from build123d import *

# Parameters (mm, degrees)
SKETCH1_W           = 105
SKETCH1_H           = 60
BOSS_EXTRUDE1_DEPTH = 15
SHELL1_T            = 2.5
FILLET1_R           = 2.5
SKETCH3_R           = 1.5
BOSS_EXTRUDE2_DEPTH = 3
SKETCH4_W           = 2
SKETCH4_H           = 60
BOSS_EXTRUDE3_DEPTH = 10
BOSS_EXTRUDE4_DEPTH = 6
SKETCH7_W           = 9
SKETCH7_H           = 10
CUT_EXTRUDE1_DEPTH  = 2.5


with BuildPart() as part:
    # Sketch1 → Boss-Extrude1 (new body)
    with BuildSketch(Plane(origin=(0, 0, 0), x_dir=(1, 0, 0), z_dir=(0, 1, 0))):
        Rectangle(SKETCH1_W, SKETCH1_H)
    extrude(amount=BOSS_EXTRUDE1_DEPTH)

    # Shell1
    shell1_openings = [part.faces().sort_by_distance(p)[0] for p in [
        (0, 15, 0),
    ]]
    offset(amount=SHELL1_T, openings=shell1_openings, kind=Kind.INTERSECTION)

    # Fillet1
    # the kernel refuses this fillet: 2.5 mm, written as the material it takes off along each edge
    with BuildSketch(Plane(origin=(52.5, 0, -30), x_dir=(1, 0, 0), z_dir=(0, 0, -1))) as fillet1_piece_1_section:
        Polygon((0, 0), (FILLET1_R, 0), (FILLET1_R, FILLET1_R), (0, FILLET1_R), align=None)
    fillet1_piece_1 = extrude(amount=FILLET1_R, mode=Mode.PRIVATE)
    fillet1_piece_1 = fillet1_piece_1 - Plane(origin=(52.5, 0, -30), x_dir=(-0.7071067811865475, 0.7071067811865475, 0), z_dir=(0, 0, -1)) * Sphere(FILLET1_R, mode=Mode.PRIVATE)
    add(fillet1_piece_1, mode=Mode.SUBTRACT)
    with BuildSketch(Plane(origin=(-52.5, 0, -30), x_dir=(0, -1, 0), z_dir=(0, 0, -1))) as fillet1_piece_2_section:
        Polygon((0, 0), (FILLET1_R, 0), (FILLET1_R, FILLET1_R), (0, FILLET1_R), align=None)
    fillet1_piece_2 = extrude(amount=FILLET1_R, mode=Mode.PRIVATE)
    fillet1_piece_2 = fillet1_piece_2 - Plane(origin=(-52.5, 0, -30), x_dir=(0.7071067811865475, 0.7071067811865475, 0), z_dir=(0, 0, -1)) * Sphere(FILLET1_R, mode=Mode.PRIVATE)
    add(fillet1_piece_2, mode=Mode.SUBTRACT)
    with BuildSketch(Plane(origin=(52.5, 0, 30), x_dir=(0, -1, 0), z_dir=(1, 0, 0))) as fillet1_piece_3_section:
        Polygon((0, 0), (FILLET1_R, 0), (FILLET1_R, -FILLET1_R), (0, -FILLET1_R), align=None)
    fillet1_piece_3 = extrude(amount=FILLET1_R, mode=Mode.PRIVATE)
    fillet1_piece_3 = fillet1_piece_3 - Plane(origin=(52.5, 0, 30), x_dir=(0, 0.7071067811865475, -0.7071067811865475), z_dir=(1, 0, 0)) * Sphere(FILLET1_R, mode=Mode.PRIVATE)
    add(fillet1_piece_3, mode=Mode.SUBTRACT)
    with BuildSketch(Plane(origin=(-52.5, 0, 30), x_dir=(0, 0, 1), z_dir=(0, -1, 0))) as fillet1_piece_4_section:
        Polygon((0, 0), (FILLET1_R, 0), (FILLET1_R, FILLET1_R), (0, FILLET1_R), align=None)
    fillet1_piece_4 = extrude(amount=FILLET1_R, mode=Mode.PRIVATE)
    fillet1_piece_4 = fillet1_piece_4 - Plane(origin=(-52.5, 0, 30), x_dir=(0.7071067811865475, 0, -0.7071067811865476), z_dir=(0, -1, 0)) * Sphere(FILLET1_R, mode=Mode.PRIVATE)
    add(fillet1_piece_4, mode=Mode.SUBTRACT)
    with BuildSketch(Plane(origin=(52.5, -2.5, -32.5), x_dir=(0, 1, 0), z_dir=(-1, 0, 0)), Plane(origin=(-52.5, -2.5, 32.5), x_dir=(0, 1, 0), z_dir=(1, 0, 0))) as fillet1_piece_5:
        with BuildLine():
            CenterArc((FILLET1_R, -FILLET1_R), FILLET1_R, 90, 90)
            Line((0, -FILLET1_R), (0, 0))
            Line((0, 0), (FILLET1_R, 0))
        make_face()
    extrude(amount=105, mode=Mode.SUBTRACT)
    with BuildSketch(Plane(origin=(55, -2.5, 30), x_dir=(0, 1, 0), z_dir=(0, 0, -1)), Plane(origin=(-55, -2.5, -30), x_dir=(0, 1, 0), z_dir=(0, 0, 1))) as fillet1_piece_6:
        with BuildLine():
            CenterArc((FILLET1_R, -FILLET1_R), FILLET1_R, 90, 90)
            Line((0, -FILLET1_R), (0, 0))
            Line((0, 0), (FILLET1_R, 0))
        make_face()
    extrude(amount=60, mode=Mode.SUBTRACT)
    with BuildSketch(Plane(origin=(-55, 21.25, -32.5), x_dir=(0, 0, 1), z_dir=(0, -1, 0)), Plane(origin=(55, 21.25, -32.5), x_dir=(-1, 0, 0), z_dir=(0, -1, 0)), Plane(origin=(55, 0, 32.5), x_dir=(-1, 0, 0), z_dir=(0, 1, 0)), Plane(origin=(-55, 21.25, 32.5), x_dir=(1, 0, 0), z_dir=(0, -1, 0))) as fillet1_piece_7:
        with BuildLine():
            CenterArc((FILLET1_R, -FILLET1_R), FILLET1_R, 90, 90)
            Line((0, -FILLET1_R), (0, 0))
            Line((0, 0), (FILLET1_R, 0))
        make_face()
    extrude(amount=21.25, mode=Mode.SUBTRACT)

    # Sketch3 → Boss-Extrude2 (add)
    # profile 1 of 2: a face of its own
    with BuildSketch(Plane(origin=(0, 15, 0), x_dir=(1, 0, 0), z_dir=(0, 1, 0))):
        with BuildLine():
            Line((55, 5), (55, -5))
            ThreePointArc((55, -5), (60, 0), (55, 5))
        make_face()
        with Locations(Location((57.5, 0, 0), (0, 0, 270))):
            Circle(SKETCH3_R, mode=Mode.SUBTRACT)
    # profile 2 of 2: a face of its own
    with BuildSketch(Plane(origin=(0, 15, 0), x_dir=(1, 0, 0), z_dir=(0, 1, 0))):
        with BuildLine():
            ThreePointArc((-55, 5), (-60, 0), (-55, -5))
            Line((-55, -5), (-55, 5))
        make_face()
        with Locations(Location((-57.5, 0, 0), (0, 0, 270))):
            Circle(SKETCH3_R, mode=Mode.SUBTRACT)
    extrude(amount=-BOSS_EXTRUDE2_DEPTH)

    # Sketch4 → Boss-Extrude3 (add)
    with BuildSketch(Plane(origin=(0, 0, 0), x_dir=(1, 0, 0), z_dir=(0, 1, 0))):
        with Locations((-33.5, 0)):
            Rectangle(SKETCH4_W, SKETCH4_H)
    extrude(amount=BOSS_EXTRUDE3_DEPTH)

    # Sketch5 → Boss-Extrude4 (add)
    with BuildSketch(Plane.ZY.offset(55)):
        with BuildLine():
            Line((-27, 9), (-27, 1))
            Line((-27, 1), (-16, 1))
            Line((-16, 1), (-16, 9))
            Line((-16, 9), (-16.601020514, 9))
            ThreePointArc((-16.601020514, 9), (-21.5, 13), (-26.398979486, 9))
            Line((-26.398979486, 9), (-27, 9))
        make_face()
        with BuildLine():
            Line((-17.5, 8), (-17, 8))
            Line((-17, 8), (-17, 2))
            Line((-17, 2), (-26, 2))
            Line((-26, 2), (-26, 8))
            Line((-26, 8), (-25.5, 8))
            ThreePointArc((-25.5, 8), (-21.5, 12), (-17.5, 8))
        make_face(mode=Mode.SUBTRACT)
    extrude(amount=-BOSS_EXTRUDE4_DEPTH)

    # Sketch7 → Cut-Extrude1 (cut)
    with BuildSketch(Plane.ZY.offset(55)):
        with Locations((-21.5, 7)):
            Rectangle(SKETCH7_W, SKETCH7_H)
    extrude(amount=-CUT_EXTRUDE1_DEPTH, mode=Mode.SUBTRACT)


solid = part.part
Work out the finished part from the listing and answer in its coordinate system (mm). A direction names the side the tool comes from. Round coordinates to 2 decimals unless told otherwise and drop trailing zeros. Write each loop counter-clockwise with the first axis right and the second up, starting at its lowest first coordinate (ties: lowest second). Pieces come first, ordered by that corner, then holes. Notation, with made-up numbers: (65.25, 35.5) -> (89.25, 35.5) arc R16 ccw to (89.25, 58.5) -> close; hole circle Ø10 at (2, 41). An arc over 180 degrees is marked (long way). Write each question's results on one line, items separated by ' | '.
Item 1: A cutting plane is placed at D-D, the plane x = 18.5. Determine the outline of the cut face in (y, z), plus the area to 3 significant figures.
Result set:
outline: (-2.5, -30) arc R2.5 ccw to (0, -32.5) -> (15, -32.5) -> (15, -30) -> (0, -30) -> (0, 30) -> (15, 30) -> (15, 32.5) -> (0, 32.5) arc R2.5 ccw to (-2.5, 30) -> close | area: 235 mm^2
Item 2: Flat-ended cylindrical pins translate along their axes: P1, Ø6, axis at y = 9.5, z = -22, coming from the +X side; P2, Ø10, axis at x = -7, z = 2.5, coming from the +Y side; P3, Ø3, axis at y = 10.5, z = -25, coming from the -X side; P4, Ø1.8, axis at x = -57.5, z = 0, coming from the -Y side. Find the tip coordinate at first contact, or state that the pin passes through.
Result set:
P1: x = 55 | P2: y = 0 | P3: x = -55 | P4: through
Item 3: A cutting plane is placed at B-B, the plane x = 57.5. Determine the outline of the cut face in (y, z), plus the area to 3 significant figures.
Result set:
outline: (12, -4.33) -> (15, -4.33) -> (15, -1.5) -> (12, -1.5) -> close; (12, 1.5) -> (15, 1.5) -> (15, 4.33) -> (12, 4.33) -> close | area: 17.0 mm^2
Item 4: Find the intervals of material crossed by line 1 along X through (y, z) = (5, 16.5); line 2 along Z through (x, y) = (-26, 12.75); line 3 along X through (y, z) = (13.65, 0), in increasing order. Write a range as [from, to].
Result set:
line 1: [-55, -52.5], [-34.5, -32.5], [52.5, 55] | line 2: [-32.5, -30], [30, 32.5] | line 3: [-60, -59], [-56, -52.5], [52.5, 56], [59, 60]
Item 5: A cutting plane is placed at A-A, the plane y = 4.5. Determine the outline of the cut face in (x, z), plus the area to 3 significant figures.
Result set:
outline: (-55, -30) arc R2.5 ccw to (-52.5, -32.5) -> (52.5, -32.5) arc R2.5 ccw to (55, -30) -> (55, 30) arc R2.5 ccw to (52.5, 32.5) -> (-52.5, 32.5) arc R2.5 ccw to (-55, 30) -> (-55, -17) -> (-49, -17) -> (-49, -16) -> (-52.5, -16) -> (-52.5, 30) -> (-34.5, 30) -> (-34.5, -30) -> (-52.5, -30) -> (-52.5, -27) -> (-49, -27) -> (-49, -26) -> (-55, -26) -> close; hole (-32.5, -30) -> (52.5, -30) -> (52.5, 30) -> (-32.5, 30) -> close | area: 949 mm^2
Item 6: The mould has two halves that part along Y. Classify faces 5 (the face through (54, 8, -32)), 6 (the face through (-51, 1, -22)), 7 (the face through (-50.8, 13, -21.4)), 8 (the face through (-56, 12, -1)): +Y half, -Y half, draft (parallel to the pull), parting line (faces both ways), or undercut.
Result set:
face 5: draft | face 6: undercut | face 7: +Y half | face 8: -Y half
Item 7: Which of the six approach directions +Z, -Z, +X, -X, +Y, -Y give full straight-line access (tool end or side, diameter ignored) to faces 1 (the face through (-54, -2, 0)), 2 (the face through (55.8, 12, -0.1)), 3 (the face through (-32.5, 5, 0)), 4 (the face through (-53, 6, -17))?
Result set:
face 1: +Z, -Z, -X, -Y | face 2: +Z, -Z, +X, -Y | face 3: +Y | face 4: -X
Item 8: A cutting plane is placed at C-C, the plane z = -10.5. Determine the outline of the cut face in (x, y).
Result set:
outline: (-55, 0) arc R2.5 ccw to (-52.5, -2.5) -> (52.5, -2.5) arc R2.5 ccw to (55, 0) -> (55, 15) -> (52.5, 15) -> (52.5, 0) -> (-32.5, 0) -> (-32.5, 10) -> (-34.5, 10) -> (-34.5, 0) -> (-52.5, 0) -> (-52.5, 15) -> (-55, 15) -> close
